from build123d import *

# Parameters (mm, degrees)
SKETCH1_R           = 45
BOSS_EXTRUDE1_DEPTH = 2
CUT_EXTRUDE2_DEPTH  = 64.671029519
CIRPATTERN1_COUNT   = 32
SKETCH4_R           = 10
CUT_EXTRUDE3_DEPTH  = 10


with BuildPart() as part:
    # Sketch1 → Boss-Extrude1 (new body)
    with BuildSketch(Plane(origin=(0, 0, 0), x_dir=(0, 0, -1), z_dir=(1, 0, 0))):
        Circle(SKETCH1_R)
    extrude(amount=BOSS_EXTRUDE1_DEPTH)

    # Sketch3 → Cut-Extrude2 (cut, symmetric)
    with BuildSketch(Plane(origin=(2, 0, 0), x_dir=(0, 0, -1), z_dir=(1, 0, 0))):
        Polygon((111.061055433, 234.770812069), (0, 45), (-4.384441822, 37.508273204), (-11.303681047, 43.557166974), (-176.845255951, 188.275880779), (-246.955404965, 622.412545429), (40.950906418, 668.907476719), align=None)
    cut_extrude2 = extrude(amount=CUT_EXTRUDE2_DEPTH, both=True, mode=Mode.SUBTRACT)

    # CirPattern1: Cut-Extrude2 ×32 about axis
    cirpattern1_axis = Axis((2, 0, 0), (-1, 0, 0))
    for i in range(1, CIRPATTERN1_COUNT):
        add(cut_extrude2.rotate(cirpattern1_axis, i * 360 / CIRPATTERN1_COUNT), mode=Mode.SUBTRACT)

    # Sketch4 → Cut-Extrude3 (cut)
    with BuildSketch(Plane(origin=(2, 0, 0), x_dir=(0, 0, -1), z_dir=(1, 0, 0))):
        Circle(SKETCH4_R)
    extrude(amount=-CUT_EXTRUDE3_DEPTH, mode=Mode.SUBTRACT)


solid = part.part
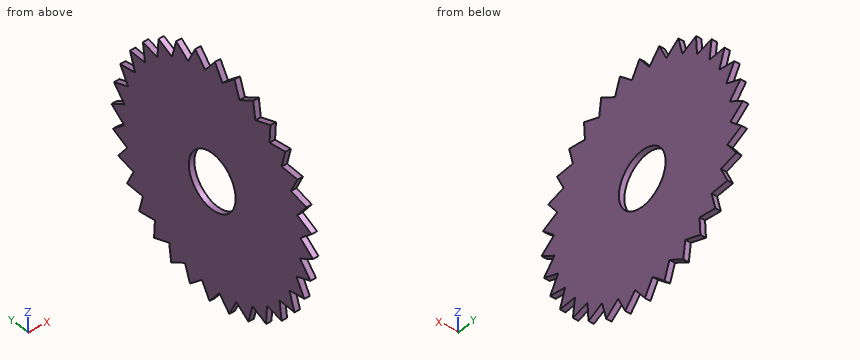
Build history of the part. All positions in model axes, mm. Coordinates: 2 decimals unless noted, no trailing zeros. Write each loop counter-clockwise with the first axis right and the second up, starting at its lowest first coordinate (ties: lowest second). Pieces come first, ordered by that corner, then holes. Notation, with made-up numbers: (-14.75, 71.5) -> (13.25, 71.5) arc R7 cw to (13.25, 84.5) -> close; hole circle Ø8 at (-12.5, 22). An arc over 180 degrees is marked (long way). Use CSV: the item, a comma, the result in double quotes. Start each with the question number.
Q1. Cut at B-B, the plane z = 0. List the corners of the cut face in (x, y).
Q2. Drill centre lines: probe 1 along Z at (x, y) = (0.6, 39); probe 2 along Y at (x, z) = (0.85, 36.5); probe 3 along Y at (x, z) = (1.95, 39.5). Where is each one in solid material? Low to high.
Q3. Cut at A-A, the plane y = 5.5. List the corners of the cut face in (x, z), then the cut area to 3 significant figures.
Q4. Flat gauge pin, fed straight in: pin 1 Ø4 at (y, z) = (-25, 33) entering from +X. Where does the tip first touch, or does it go through?
Q5. Cut at C-C, the plane y = -26. List the corners of the cut face in (x, z).
Q6. Cut at D-D, the plane y = 26.5. List the corners of the cut face in (x, z).
Checked values:
1,outline,"(0, -41.56) -> (2, -41.56) -> (2, -10) -> (0, -10) -> close; (0, 10) -> (2, 10) -> (2, 41.56) -> (0, 41.56) -> close"
2,probe 1,"z = -15.74 to -13.82, -8.98 to -4.22, -1.97 to 3.51, 6.09 to 10.56, 16.95 to 17.58"
2,probe 2,"y = -17.92 to -12.6, -11.42 to 10.22, 10.53 to 16.42"
2,probe 3,"y = -10.38 to -6.66, -3.22 to 1.59, 4.67 to 8.73, 14.48 to 15.61"
3,outline,"(0, -38.48) -> (2, -38.48) -> (2, -8.35) -> (0, -8.35) -> close; (0, 8.35) -> (2, 8.35) -> (2, 40.44) -> (0, 40.44) -> close"
3,area,"124 mm²"
4,pin 1,"stops at x = 2"
5,outline,"(0, -30.3) -> (2, -30.3) -> (2, 28.95) -> (0, 28.95) -> close"
6,outline,"(0, -29.01) -> (2, -29.01) -> (2, 30.43) -> (0, 30.43) -> close"
